from build123d import *

# Parameters (mm, degrees)
EXTRUDE_1_DEPTH     = 25
RIB_1_REACH         = 53.701
SKETCH_3_WALL_W     = 143.585893822
SKETCH_3_WALL_H     = 3
FILLET_1_R          = 2
CUT_EXTRUDE_1_DEPTH = 3
CUT_EXTRUDE_2_DEPTH = 3
SKETCH_7_R          = 1.65
CUT_EXTRUDE_3_DEPTH = 11
SKETCH_6_R          = 1.65
CUT_EXTRUDE_4_DEPTH = 11


with BuildPart() as part:
    # Эскиз1 → Бобышка-Вытянуть1 (new body)
    with BuildSketch(Plane.XY):
        Polygon((0, 0), (-32, 0), (-32, 5), (-5, 5), (-5, 32), (0, 32), align=None)
    extrude(amount=EXTRUDE_1_DEPTH)

    # Эскиз3 wall → Ребро1 (add, up to next)
    with BuildSketch(Plane(origin=(-18.5, 18.5, 25), x_dir=(0.707106781187, 0.707106781187, 0), z_dir=(-0.707106781187, 0.707106781187, 0)), mode=Mode.PRIVATE) as rib_1_sk1:
        with Locations((0, 1.5)):
            Rectangle(SKETCH_3_WALL_W, SKETCH_3_WALL_H)
    rib_1_tool1 = extrude(rib_1_sk1.sketch, amount=-RIB_1_REACH, mode=Mode.PRIVATE) - part.part
    rib_1 = rib_1_tool1.solids().sort_by_distance((-18.5, 18.5, 25))[0]
    add(rib_1)

    # Зеркальное отражение1: Ребро1 across plane
    add(rib_1.mirror(Plane.XY.offset(12.5)))

    # Скругление1
    fillet_1_edges = [part.edges().sort_by_distance(p)[0] for p in [
        (-32, 2.5, 25),
        (-32, 2.5, 0),
        (-2.5, 32, 0),
        (-2.5, 32, 25),
    ]]
    fillet(fillet_1_edges, radius=FILLET_1_R)

    # Эскиз4 → Вырез-Вытянуть1 (cut)
    with BuildSketch(Plane(origin=(0, 5, 0), x_dir=(1, 0, 0), z_dir=(0, 1, 0))):
        Polygon((-15.035898385, -12.5), (-16.767949192, -9.5), (-20.232050808, -9.5), (-21.964101615, -12.5), (-20.232050808, -15.5), (-16.767949192, -15.5), align=None)
    extrude(amount=-CUT_EXTRUDE_1_DEPTH, mode=Mode.SUBTRACT)

    # Эскиз5 → Вырез-Вытянуть2 (cut)
    with BuildSketch(Plane.ZY.offset(5)):
        Polygon((12.5, 15.035898385), (15.5, 16.767949192), (15.5, 20.232050808), (12.5, 21.964101615), (9.5, 20.232050808), (9.5, 16.767949192), align=None)
    extrude(amount=-CUT_EXTRUDE_2_DEPTH, mode=Mode.SUBTRACT)

    # Эскиз7 → Вырез-Вытянуть3 (cut)
    with BuildSketch(Plane.ZY.offset(2)):
        with Locations((12.5, 18.5)):
            Circle(SKETCH_7_R)
    extrude(amount=-CUT_EXTRUDE_3_DEPTH, mode=Mode.SUBTRACT)

    # Эскиз6 → Вырез-Вытянуть4 (cut)
    with BuildSketch(Plane(origin=(0, 2, 0), x_dir=(1, 0, 0), z_dir=(0, 1, 0))):
        with Locations(Location((-18.5, -12.5, 0), (0, 0, 270))):
            Circle(SKETCH_6_R)
    extrude(amount=-CUT_EXTRUDE_4_DEPTH, mode=Mode.SUBTRACT)


solid = part.part
Source: CAD feature listing. Evaluate the final solid. Frame: model axes, mm. A direction names the side the tool comes from. Round coordinates to 2 decimals unless told otherwise and drop trailing zeros. Loops run counter-clockwise (first coordinate to the right, second up) from the corner with the lowest first, then second, coordinate; pieces in that order, holes last. Notation, with made-up numbers: (-36, -8) - (4, -8) arc R32 ccw to (4, 28) - close; hole circle Ø2 at (71.25, -10.5). An arc over 180 degrees is marked (long way). Write item = value, one per line. Start each with the question number.
Item 1: Material intervals for line 1 (Z direction, x = -15.5, y = 7.5); line 2 (Y direction, x = -1.35, z = 12.5); line 3 (X direction, y = 1.35, z = 12.5), sorted ascending.
Item 2: Mould query, pull axis X, two halves, no side actions, for faces 6 (the face through (-2, 17, 11)), 7 (the face through (-15.9, 3.5, 14)), 8 (the face through (-22, 5, 14)). Classes: released by +X, released by -X, zero draft, split by the parting line, or undercut.
Item 3: Section query C-C on x = -28. Output: boundary loops of the cut face in (y, z), plus the area to 3 significant figures.
Item 4: Reachability of faces 1 (the face through (-31.43, 2.77, 0.6)), 2 (the face through (-19, 4, 15.5)), 3 (the face through (-32, 2, 12)), 4 (the face through (-3.5, 21.1, 11)), 5 (the face through (-5, 15, 14)) from +Z, -Z, +X, -X, +Y, -Y: full face, straight path, thin tool, end or side. Return the list, or none.
Item 5: Section query B-B on x = -18.5. Output: boundary loops of the cut face in (y, z), plus the area to 3 significant figures.
Item 6: Section query D-D on z = 22.5. Output: boundary loops of the cut face in (x, y).
Item 7: First-contact query: pin 1 Ø3 at (x, z) = (-20, 13) entering from +Y; pin 2 Ø3 at (y, z) = (17.5, 14.5) entering from -X; pin 3 Ø4 at (x, z) = (-18.5, 12.5) entering from +Y; pin 4 Ø3 at (y, z) = (18.5, 12.5) entering from +X. Flat tips, straight axial feed; report the tip coordinate or a pass-through.
Item 8: Section query A-A on y = 18.5. Output: boundary loops of the cut face in (x, z).
Results list:
q1.line_1 = 0 to 3, 22 to 25
q1.line_2 = 0 to 16.85, 20.15 to 32
q1.line_3 = -32 to -20.15, -16.85 to 0
q2.face_6 = released by -X
q2.face_7 = undercut
q2.face_8 = zero draft
q3.outline = (0, 0) - (9, 0) - (9, 3) - (5, 3) - (5, 22) - (9, 22) - (9, 25) - (0, 25) - close
q3.area = 149 mm²
q4.face_1 = -Z, -X, +Y, -Y
q4.face_2 = +Y
q4.face_3 = +Z, -Z, -X, +Y, -Y
q4.face_4 = -X
q4.face_5 = -X, +Y
q5.outline = (0, 0) - (18.5, 0) - (18.5, 3) - (5, 3) - (5, 9.5) - (2, 9.5) - (2, 10.85) - (0, 10.85) - close; (0, 14.15) - (2, 14.15) - (2, 15.5) - (5, 15.5) - (5, 22) - (18.5, 22) - (18.5, 25) - (0, 25) - close
q5.area = 181 mm²
q6.outline = (-32, 0) - (0, 0) - (0, 32) - (-5, 32) - (-32, 5) - close
q7.pin_1 = 5
q7.pin_2 = -5
q7.pin_3 = 2
q7.pin_4 = through
q8.outline = (-18.5, 0) - (0, 0) - (0, 10.85) - (-2, 10.85) - (-2, 9.5) - (-5, 9.5) - (-5, 3) - (-18.5, 3) - close; (-18.5, 22) - (-5, 22) - (-5, 15.5) - (-2, 15.5) - (-2, 14.15) - (0, 14.15) - (0, 25) - (-18.5, 25) - close
